Source: three-view drawing plus pictorial views. Frame: mm from the lowest corner of the part. A direction names the side the tool comes from. Round coordinates to 2 decimals unless told otherwise and drop trailing zeros. Order: outer loops, then holes, each group sorted by start corner. A loop starts at its lowest first (then second) coordinate and runs counter-clockwise, first axis right, second up. Notation, with made-up numbers: (23, 63) -> (74, 63) arc R13 ccw to (74, 67) -> close; hole circle Ø3 at (17.25, 32.5). An arc over 180 degrees is marked (long way). Answer as CSV lines item,"result".
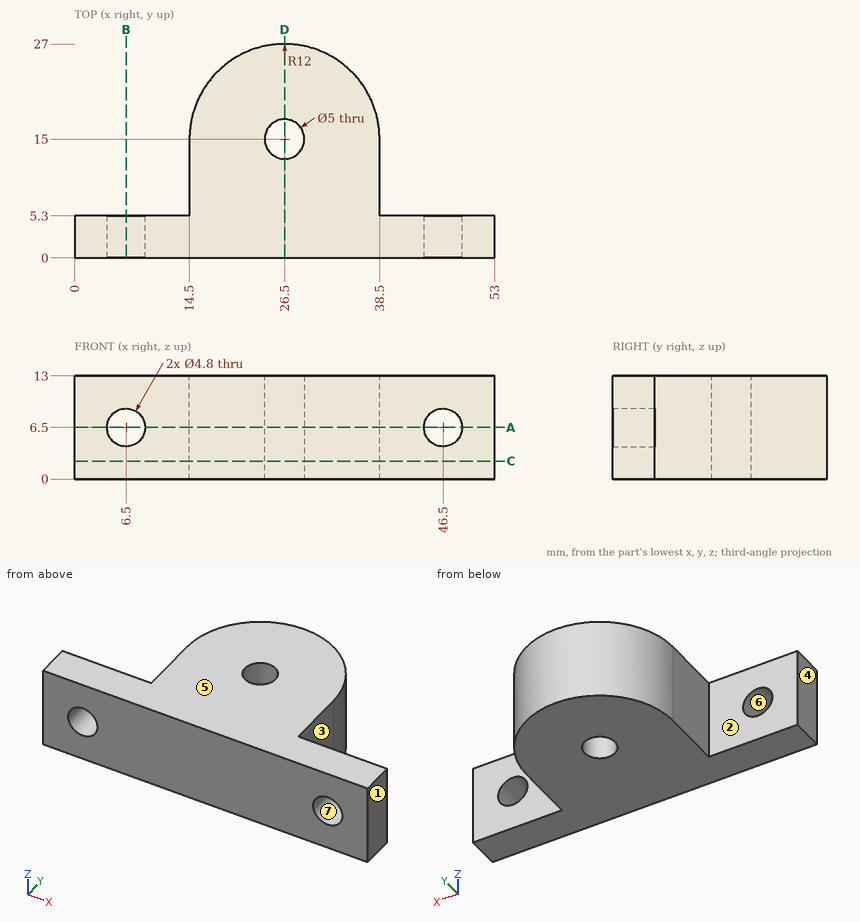
1. Line query: L1, parallel to Y at x = 26.5, z = 8.5; L2, parallel to Z at x = 6.5, y = 1.5; L3, parallel to Y at x = 8.5, z = 1.75. Output: solid intervals per line, ascending. Write a range as [from, to].
Results below:
L1,"[0, 12.5], [17.5, 27]"
L2,"[0, 4.1], [8.9, 13]"
L3,"[0, 5.3]"
2. Section query D-D on x = 26.5. Return loops of the section in (y, z).
Results below:
outline,"(0, 0) -> (12.5, 0) -> (12.5, 13) -> (0, 13) -> close; (17.5, 0) -> (27, 0) -> (27, 13) -> (17.5, 13) -> close"
3. Mould query, pull axis X, two halves, no side actions, for the marked faces 4, 5, 6 and 7. Classes: released by +X, released by -X, zero draft, split by the parting line, or undercut.
Results below:
face 4,"released by -X"
face 5,"zero draft"
face 6,"undercut"
face 7,"undercut"
4. Section query A-A on z = 6.5. Return loops of the section in (x, y).
Results below:
outline,"(0, 0) -> (4.1, 0) -> (4.1, 5.3) -> (0, 5.3) -> close; (8.9, 0) -> (44.1, 0) -> (44.1, 5.3) -> (38.5, 5.3) -> (38.5, 15) arc R12 ccw to (14.5, 15) -> (14.5, 5.3) -> (8.9, 5.3) -> close; (48.9, 0) -> (53, 0) -> (53, 5.3) -> (48.9, 5.3) -> close; hole circle Ø5 at (26.5, 15)"
5. Reachability of the marked faces 1, 2 and 3 from +Z, -Z, +X, -X, +Y, -Y: full face, straight path, thin tool, end or side. Return the list, or none.
Results below:
face 1,"+Z, -Z, +X, +Y, -Y"
face 2,"+Z, -Z, -X, +Y"
face 3,"+Z, -Z, +X, +Y"
6. Section query B-B on x = 6.5. Return loops of the section in (y, z), and give its area (3 significant figures).
Results below:
outline,"(0, 0) -> (5.3, 0) -> (5.3, 4.1) -> (0, 4.1) -> close; (0, 8.9) -> (5.3, 8.9) -> (5.3, 13) -> (0, 13) -> close"
area,"43.5 mm2"
7. Pin query (flat end, axial travel): pin 1 (6.5 mm diameter, centred on x = 5.5, z = 8.5, fed in from +Y); pin 2 (3 mm diameter, centred on x = 12.5, z = 3.5, fed in from -Y); pin 3 (1.5 mm diameter, centred on x = 20, z = 3, fed in from +Y); pin 4 (1 mm diameter, centred on x = 30.5, z = 5, fed in from +Y). Return the tip coordinate at first contact, or that it passes through.
Results below:
pin 1,"y = 5.3"
pin 2,"y = 0"
pin 3,"y = 25.53"
pin 4,"y = 26.48"
8. Section query C-C on z = 2.25. Return loops of the section in (x, y), and give its area (3 significant figures).
Results below:
outline,"(0, 0) -> (53, 0) -> (53, 5.3) -> (38.5, 5.3) -> (38.5, 15) arc R12 ccw to (14.5, 15) -> (14.5, 5.3) -> (0, 5.3) -> close; hole circle Ø5 at (26.5, 15)"
area,"720 mm2"
